from build123d import *

# Parameters (mm, degrees)
F0_W     = 40
F0_H     = 15
F1_DEPTH = 25
F2_DEPTH = 2
F3_R     = 2.5
F4_DEPTH = 5


with BuildPart() as f1:
    # F0 (on Front) → F1 (new body)
    with BuildSketch(Plane.XZ):
        with BuildLine():
            Line((-20, -8.5), (20, -8.5))
            ThreePointArc((20, -8.5), (20.707107, -8.207107), (21, -7.5))
            Line((21, -7.5), (21, 7.5))
            ThreePointArc((21, 7.5), (20.707107, 8.207107), (20, 8.5))
            Line((20, 8.5), (-20, 8.5))
            ThreePointArc((-20, 8.5), (-20.707107, 8.207107), (-21, 7.5))
            Line((-21, 7.5), (-21, -7.5))
            ThreePointArc((-21, -7.5), (-20.707107, -8.207107), (-20, -8.5))
        make_face()
        Rectangle(F0_W, F0_H, mode=Mode.SUBTRACT)
    extrude(amount=F1_DEPTH)

    # F0 (on Front) → F2 (join)
    with BuildSketch(Plane.XZ):
        Rectangle(F0_W, F0_H)
    extrude(amount=F2_DEPTH)

    # F3 (on face) → F4 (cut)
    with BuildSketch(Plane.YZ.offset(21)):
        with Locations((-12.5, 0)):
            Circle(F3_R)
    extrude(amount=-F4_DEPTH, mode=Mode.SUBTRACT)


solid = f1.part
Geometry: final body of the model. Coordinates: model frame, mm. A direction names the side the tool comes from. Round coordinates to 2 decimals unless told otherwise and drop trailing zeros. Loops run counter-clockwise (first coordinate to the right, second up) from the corner with the lowest first, then second, coordinate; pieces in that order, holes last. Notation, with made-up numbers: (68, -32) -> (84, -32) arc R14 cw to (84, -23) -> close; hole circle Ø11 at (-28, 36). An arc over 180 degrees is marked (long way). One line per question, with ' | ' between items. Start each with the question number.
1. Contact query for a flat-ended pin moving along its axis: pin 1 (3 mm diameter, centred on y = -12.5, z = 0, fed in from +X). Output: stop coordinate, or through.
2. Section C-C on y = -10.5. Output: boundary loops of the cut face in (x, z).
3. Section B-B on y = -20.5. Output: boundary loops of the cut face in (x, z).
4. Section A-A on z = 0. Output: boundary loops of the cut face in (x, y), and give its area (3 significant figures).
5. Mould query, pull axis Z, two halves, no side actions, for faces 1 (the face through (21, -9.5, -0.1)), 2 (the face through (20.699, -12.325, -8.215)), 3 (the face through (0, -13, -7.5)). Classes: pulls with the +Z half, pulls with the -Z half, needs draft (parallel to the pull), parting line crosses it, or undercut.
6. Line query: line 1 along Z through (x, y) = (-11, -3); line 2 along X through (y, z) = (-20, 5.25); line 3 along Y through (x, z) = (6, -3). Output: solid intervals per line, ascending. Write a range as [from, to].
7. Section D-D on x = -8.5. Output: boundary loops of the cut face in (y, z).
8. Set-up query: faces 4 (the face through (20.5, -15, 0.1)), 5 (the face through (-21, -12, 0)), 6 (the face through (20, -16, 0)). Return all of +Z, -Z, +X, -X, +Y, -Y with unobstructed straight access to the full face (end or side cutting, diameter ignored); none if empty.
Returned:
1) pin 1: stops at x = -20
2) outline: (-21, -7.5) arc R1 ccw to (-20, -8.5) -> (20, -8.5) arc R1 ccw to (21, -7.5) -> (21, -1.5) -> (20, -1.5) -> (20, -7.5) -> (-20, -7.5) -> (-20, 7.5) -> (20, 7.5) -> (20, 1.5) -> (21, 1.5) -> (21, 7.5) arc R1 ccw to (20, 8.5) -> (-20, 8.5) arc R1 ccw to (-21, 7.5) -> close
3) outline: (-21, -7.5) arc R1 ccw to (-20, -8.5) -> (20, -8.5) arc R1 ccw to (21, -7.5) -> (21, 7.5) arc R1 ccw to (20, 8.5) -> (-20, 8.5) arc R1 ccw to (-21, 7.5) -> close; hole (-20, -7.5) -> (20, -7.5) -> (20, 7.5) -> (-20, 7.5) -> close
4) outline: (-21, -25) -> (-20, -25) -> (-20, -2) -> (20, -2) -> (20, -10) -> (21, -10) -> (21, 0) -> (-21, 0) -> close; (20, -25) -> (21, -25) -> (21, -15) -> (20, -15) -> close | area: 125 mm2
5) face 1: needs draft | face 2: pulls with the -Z half | face 3: undercut
6) line 1: z = [-8.5, -7.5], [7.5, 8.5] | line 2: x = [-21, -20], [20, 21] | line 3: y = [-2, 0]
7) outline: (-25, -8.5) -> (0, -8.5) -> (0, 8.5) -> (-25, 8.5) -> (-25, 7.5) -> (-2, 7.5) -> (-2, -7.5) -> (-25, -7.5) -> close
8) face 4: +X | face 5: +Z, -Z, -X, +Y, -Y | face 6: -Y
